Here's how the part is built. I have some questions about the finished solid (model axes, mm). A direction names the side the tool comes from. Round coordinates to 2 decimals unless told otherwise and drop trailing zeros. Write each loop counter-clockwise with the first axis right and the second up, starting at its lowest first coordinate (ties: lowest second). Pieces come first, ordered by that corner, then holes. Notation, with made-up numbers: (84.5, -5) - (109.5, -5) arc R7 ccw to (109.5, 1) - close; hole circle Ø2 at (26, 59.25). An arc over 180 degrees is marked (long way). Use one line per item in the form item = value. Start each with the question number.
1. If I drill on line 1 along Z through (x, y) = (10, -1.8); line 2 along X through (y, z) = (-1.75, 1.5); line 3 along X through (y, z) = (-0.8, 6.25), over which ranges is the centre line in solid material (lowest first)?
2. I want a section at A-A, the plane y = -1.55. List the corners of the cut face in (x, z) for me.
3. Which directions (+Z, -Z, +X, -X, +Y, -Y) give clear straight access to the entire face, cutting with the end or side of a thin tool? Please do faces 4 (the flat face through (-6, -1, -2)), 5 (the flat face through (36, -1, 0)), 6 (the flat face through (13.398, -1.479, -2.993)), 7 (the flat face through (20, -1, 7)).
4. I want a section at B-B, the plane x = 24.5. List the corners of the cut face in (y, z) for me, plus the area to 3 significant figures.
5. We'd pull the mould along Z, two halves only. Please class faces 1 (the flat face through (-10, -1, 0)), 2 (the flat face through (10, -1, 4)), 3 (the flat face through (23.381, -1.479, -2.535)): +Z half, -Z half, draft (parallel to the pull), parting line (faces both ways), or undercut.
6. Will these pins go through, and if not, where does the flat tip stop? pin 1 (1.5 mm diameter, centred on x = 0.5, y = -2.5, fed in from -Z); pin 2 (1 mm diameter, centred on x = 37, y = -2.5, fed in from -Z); pin 3 (1.5 mm diameter, centred on x = 11.5, y = -1.5, fed in from -Z); pin 4 (5.5 mm diameter, centred on x = 57.43, z = 3.5, fed in from -Y).
```python
from build123d import *

# Parameters (mm, degrees)
F0_R     = 3
F1_DEPTH = 3


# Not quite as in the source:
# - a feature names something its author has since deleted; it is built from what else it names


with BuildPart() as f1:
    # F0 (on Front) → F1 (new body)
    with BuildSketch(Plane.XZ):
        Polygon((-2, -2), (1.3333333333, 0), (0, 0), (0, 7), (-10, 2.5), (-10, -2), align=None)
        Polygon((14.2307692308, 0), (32, 0), (40, 0), (40, 7), (0, 7), (0, 0), (1.3333333333, 0), (8, 4), (13, 4), align=None)
        Polygon((15, -5), (32, 0), (14.2307692308, 0), (15, -2.5), (11.75, -3.5), align=None)
        with BuildLine():
            Line((40, 7), (40, 0))
            ThreePointArc((40, 0), (61.4283268073, 3.5), (40, 7))
        make_face()
        with Locations((57.4283268073, 3.5)):
            Circle(F0_R, mode=Mode.SUBTRACT)
    extrude(amount=F1_DEPTH)


solid = f1.part
```
Model answer:
q1.line_1 = 4 to 7
q1.line_2 = -10 to 3.83, 13.77 to 55.19, 59.66 to 61.24
q1.line_3 = -1.67 to 56.23, 58.63 to 61.08
q2.outline = (-10, -2) - (-2, -2) - (8, 4) - (13, 4) - (15, -2.5) - (11.75, -3.5) - (15, -5) - (32, 0) - (40, 0) arc R11 ccw (long way) to (40, 7) - (0, 7) - (-10, 2.5) - close; hole circle Ø6 at (57.43, 3.5)
q3.face_4 = -Z, -X, +Y, -Y
q3.face_5 = -Z, +Y, -Y
q3.face_6 = -X, +Y, -Y
q3.face_7 = +Z, -X, +Y, -Y
q4.outline = (-3, -2.21) - (0, -2.21) - (0, 7) - (-3, 7) - close
q4.area = 27.6 mm2
q5.face_1 = draft
q5.face_2 = undercut
q5.face_3 = -Z half
q6.pin_1 = -0.95
q6.pin_2 = 0
q6.pin_3 = -3.73
q6.pin_4 = through
